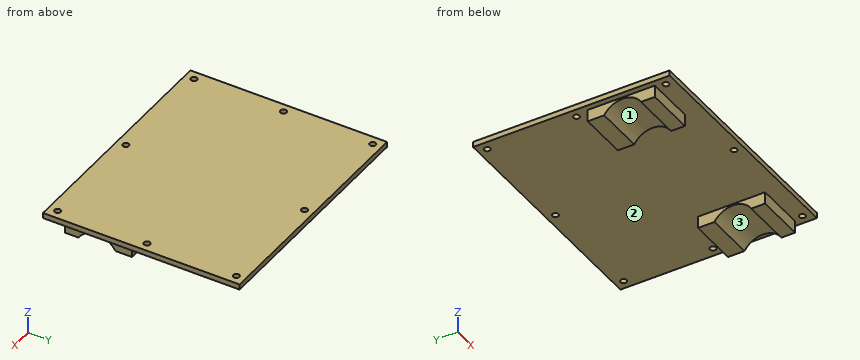
from build123d import *

# Parameters (mm, degrees)
SKETCH009_W     = 140.059471
SKETCH009_H     = 114.571171
PAD008_DEPTH    = 3.175
SKETCH013_R     = 1.778
POCKET003_DEPTH = 5.00126
SKETCH020_W     = 133.35
SKETCH020_H     = 39.116
PAD012_DEPTH    = 6.985
SKETCH021_R     = 12.49934
POCKET007_DEPTH = 136.729619
SKETCH022_W     = 76.2
SKETCH022_H     = 43.18
POCKET008_DEPTH = 8.89


with BuildPart() as part:
    # Sketch009 (on Face1 of ReferencePad006) → Pad008 (new body)
    with BuildSketch(Plane.XY.offset(25.4)):
        with Locations((0.023884, -0.09941)):
            Rectangle(SKETCH009_W, SKETCH009_H)
    extrude(amount=PAD008_DEPTH)

    # Sketch013 (on Face6 of Pad008) → Pocket003 (cut)
    with BuildSketch(Plane.XY.offset(28.575)):
        with Locations((64.782738, 52.056831)):
            Circle(SKETCH013_R)
        with Locations((64.782738, 0)):
            Circle(SKETCH013_R)
        with Locations((64.782738, -52.056831)):
            Circle(SKETCH013_R)
        with Locations((0, 52.056831)):
            Circle(SKETCH013_R)
        with Locations((-64.782738, 52.056831)):
            Circle(SKETCH013_R)
        with Locations((-64.782738, 0.043989)):
            Circle(SKETCH013_R)
        with Locations((-64.782738, -52.056831)):
            Circle(SKETCH013_R)
        with Locations((0, -52.056831)):
            Circle(SKETCH013_R)
    extrude(amount=-POCKET003_DEPTH, mode=Mode.SUBTRACT)

    # Sketch020 (on Face5 of Pad008) → Pad012 (join)
    with BuildSketch(Plane(origin=(0, 0, 25.4), x_dir=(1, 0, 0), z_dir=(0, 0, -1))):
        with Locations((0, 27.178)):
            Rectangle(SKETCH020_W, SKETCH020_H)
    extrude(amount=PAD012_DEPTH)

    # Sketch021 (on Face12 of Pad012) → Pocket007 (cut, through all)
    with BuildSketch(Plane(origin=(-66.675, 0, 0), x_dir=(0, -1, 0), z_dir=(-1, 0, 0))):
        with Locations((27.94, 11.99134)):
            Circle(SKETCH021_R)
    extrude(amount=-POCKET007_DEPTH, mode=Mode.SUBTRACT)

    # Sketch022 (on Face4 of Pocket007) → Pocket008 (cut)
    with BuildSketch(Plane(origin=(0, 0, 25.4), x_dir=(1, 0, 0), z_dir=(0, 0, -1))):
        with Locations((0, 27.94)):
            Rectangle(SKETCH022_W, SKETCH022_H)
    extrude(amount=POCKET008_DEPTH, mode=Mode.SUBTRACT)


solid = part.part
Can you work these out from the model? Positions are in its coordinate system, mm. Face numbers are marked on the shaded views. Round coordinates to 2 decimals unless told otherwise and drop trailing zeros. Write each loop counter-clockwise with the first axis right and the second up, starting at its lowest first coordinate (ties: lowest second). Pieces come first, ordered by that corner, then holes. Notation, with made-up numbers: (-0.5, 46) -> (38.5, 46) arc R23 ccw to (38.5, 66) -> close; hole circle Ø10 at (58.25, 24). An arc over 180 degrees is marked (long way). One line per question, with ' | ' between items. Start each with the question number.
1) I need wall thicknesses on line 1 (Y direction, x = 0, z = 27.3) (3 decimals); line 2 (X direction, y = -25.5, z = 25) (3 decimals); line 3 (Z direction, x = -18, y = -32) (3 decimals). Which ranges of each line are inside material? Lowest first, please. Write a range as [from, to].
2) I'm going to push flat-ended pins straight in: P1, Ø3, axis at x = 64.78, y = -52.06, coming from the -Z side; P2, Ø5.5, axis at x = 64.78, y = 52.06, coming from the -Z side; P3, Ø3.5, axis at x = 55.5, z = 22.5, coming from the +Y side; P4, Ø3.5, axis at x = -56, z = 23, coming from the -Y side. Where does each tip first touch, or does it pass through?
3) Suppose I cut it at C-C on x = 0. Write out the boundary of the cut face in (y, z) (3 decimals), then the cut area to 3 significant figures.
4) If we mould it in two halves opening along Y, with no side actions, what happens to the marked faces 1, 2 and 3? For each: released by +Y, released by -Y, zero draft, split by the parting line, or undercut.
5) Suppose I cut it at A-A on y = -12.5. Write out the boundary of the cut face in (x, z) (3 decimals), then the cut area to 3 significant figures.
6) Suppose I cut it at D-D on z = 23. Write out the boundary of the cut face in (x, y) (3 decimals).
7) Suppose I cut it at B-B on x = -60. Write out the boundary of the cut face in (y, z) (3 decimals).
Return value:
1) line 1: y = [-57.385, -53.835], [-50.279, 50.279], [53.835, 57.186] | line 2: x = [-66.675, -38.1], [38.1, 66.675] | line 3: z = [25.4, 28.575]
2) P1: passes through | P2: stops at z = 25.4 | P3: stops at y = -7.62 | P4: stops at y = -46.74
3) outline: (-57.385, 25.4) -> (-53.835, 25.4) -> (-53.835, 28.575) -> (-57.385, 28.575) -> close; (-50.279, 25.4) -> (50.279, 25.4) -> (50.279, 28.575) -> (-50.279, 28.575) -> close; (53.835, 25.4) -> (57.186, 25.4) -> (57.186, 28.575) -> (53.835, 28.575) -> close | area: 341 mm2
4) face 1: undercut | face 2: zero draft | face 3: undercut
5) outline: (-70.006, 25.4) -> (-66.675, 25.4) -> (-66.675, 18.415) -> (-38.1, 18.415) -> (-38.1, 25.4) -> (38.1, 25.4) -> (38.1, 18.415) -> (66.675, 18.415) -> (66.675, 25.4) -> (70.054, 25.4) -> (70.054, 28.575) -> (-70.006, 28.575) -> close | area: 844 mm2
6) outline: (-66.675, -46.736) -> (-38.1, -46.736) -> (-38.1, -33.86) -> (-66.675, -33.86) -> close; (-66.675, -22.02) -> (-38.1, -22.02) -> (-38.1, -7.62) -> (-66.675, -7.62) -> close; (38.1, -46.736) -> (66.675, -46.736) -> (66.675, -33.86) -> (38.1, -33.86) -> close; (38.1, -22.02) -> (66.675, -22.02) -> (66.675, -7.62) -> (38.1, -7.62) -> close
7) outline: (-57.385, 25.4) -> (-46.736, 25.4) -> (-46.736, 18.415) -> (-38.662, 18.415) arc R12.499 cw to (-17.218, 18.415) -> (-7.62, 18.415) -> (-7.62, 25.4) -> (57.186, 25.4) -> (57.186, 28.575) -> (-57.385, 28.575) -> close
